Can you work these out from the model? Positions are in its coordinate system, mm. Round coordinates to 2 decimals unless told otherwise and drop trailing zeros. Loops run counter-clockwise (first coordinate to the right, second up) from the corner with the lowest first, then second, coordinate; pieces in that order, holes last. Notation, with made-up numbers: M -40,36 L -20,36 A17 cw -20,63 Z; hole C 63.5,-18 d3. An arc over 180 degrees is marked long. Return JSON: item names as keys, results as strings.
```python
from build123d import *

# Parameters (mm, degrees)
F2_R    = 2
F3_SIZE = 1.99999


# Not quite as in the source:
# - a fillet or chamfer is up to 0.001 mm smaller than in the source, because OpenCascade refuses the exact size


with BuildPart() as f1:
    # F0 (on Front) → F1 (revolve)
    with BuildSketch(Plane.XZ):
        with BuildLine():
            Line((-13, 0), (-10.9896817121, 0))
            ThreePointArc((-10.9896817121, 0), (-9.4533501693, 8.6567410673), (-6.6803534332, 17))
            Line((-6.6803534332, 17), (0, 17))
            Line((0, 17), (0, 19))
            Line((0, 19), (-8, 19))
            ThreePointArc((-8, 19), (-11.2501561273, 9.6974095072), (-13, 0))
        make_face()
    revolve(axis=Axis((-6.5, 0, 0), (-1, 0, 0)))

    # F2
    f2_edges = [f1.edges().sort_by_distance(p)[0] for p in [
        (-8, 0, -19),
    ]]
    fillet(f2_edges, radius=F2_R)

    # F3 (size 2 in the source; OpenCascade refuses exactly that, so slightly less here)
    f3_edges = [f1.edges().sort_by_distance(p)[0] for p in [
        (0, 0, -17),
    ]]
    chamfer(f3_edges, length=F3_SIZE)


solid = f1.part
```
Q1. Thinking about a two-plate mould opening in Z: for faces 1 (the cylindrical face through (-3.387, -16.856, 8.767)), 2 (the cylindrical face through (-4.307, 14.334, 9.139)), which applies, pulls with the +Z half, pulls with the -Z half, needs draft (parallel to the pull), parting line crosses it, or undercut?
Results:
{"face 1": "parting line crosses it", "face 2": "undercut"}
Q2. I'm going to push flat-ended pins straight in: pin 1 Ø4 at (x, z) = (-6.5, 9) entering from +Y; pin 2 Ø3 at (x, z) = (-9, 12.5) entering from -Y; pin 3 Ø6 at (y, z) = (-2.5, -7) entering from +X. Where does each tip first touch, or does it pass through?
Results:
{"pin 1": "stops at y = 17.66", "pin 2": "stops at y = -14.62", "pin 3": "stops at x = -8.97"}
Q3. Suppose I cut it at A-A, the plane x = -4.75. Please give me the cut outline in (y, z), plus the area to 3 significant figures.
Results:
{"outline": "C 0,0 d38; hole C 0,0 d34", "area": "226 mm2"}
Q4. If I drill on line 1 along Y through (x, z) = (-4.45, 0); line 2 along Z through (x, y) = (-5.25, -2); line 3 along Y through (x, z) = (-1.25, 16), over which ranges is the centre line in solid material (lowest first)?
Results:
{"line 1": "y = -19 to -17, 17 to 19", "line 2": "z = -18.89 to -16.88, 16.88 to 18.89", "line 3": "y = -10.25 to -7.69, 7.69 to 10.25"}
